from build123d import *

# Parameters (mm, degrees)
F0_R     = 28.2106727932
F0_R_2   = 22.6152096398
F1_DEPTH = 101.6
F3_W     = 56.4213455863
F3_H     = 50.825882433
F4_DEPTH = 3.175


with BuildPart() as f1:
    # F0 (on Top) → F1 (new body)
    with BuildSketch(Plane.XY):
        Circle(F0_R)
        Circle(F0_R_2, mode=Mode.SUBTRACT)
    extrude(amount=F1_DEPTH)


with BuildPart() as f1_1:
    # F2: moved
    add(f1.part.moved(Location((0, 0, -50.8))))

    # F3 (on Top) → F4 (cut)
    with BuildSketch(Plane.XY):
        with Locations((0, 2.7977315767)):
            Rectangle(F3_W, F3_H)
    extrude(amount=F4_DEPTH, mode=Mode.SUBTRACT)


solid = f1_1.part
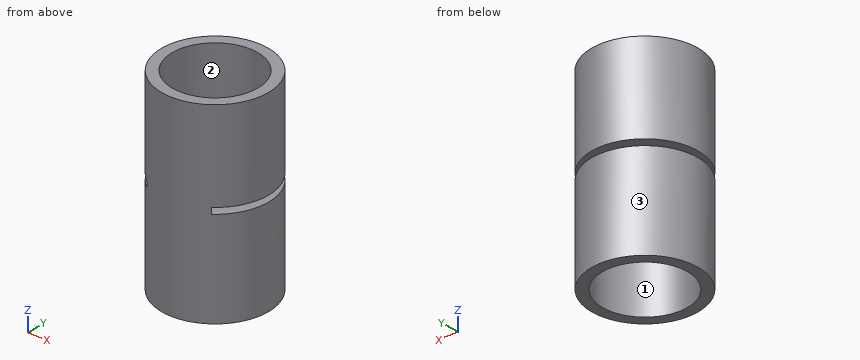
Design review of the part built by this model. Coordinates are the model's own, in mm. Face numbers are marked on the shaded views. Round coordinates to 2 decimals unless told otherwise and drop trailing zeros. Loops run counter-clockwise (first coordinate to the right, second up) from the corner with the lowest first, then second, coordinate; pieces in that order, holes last. Notation, with made-up numbers: (-1.75, 64.5) - (32.25, 64.5) arc R20 ccw to (32.25, 78.5) - close; hole circle Ø5 at (19.5, 89). An arc over 180 degrees is marked (long way). One line per item, written item: value. Start each with the question number.
1) Consider section A-A on y = 0. Give the boundary of the cut face in (x, z) (3 decimals), then the cut area to 3 significant figures.
2) Insertion check: pin 1 Ø4 at (y, z) = (-22, -9.5) entering from +X; pin 2 Ø4 at (x, z) = (-13.5, -33.5) entering from -Y; pin 3 Ø1.5 at (y, z) = (0.5, -12) entering from +X; pin 4 Ø4 at (x, y) = (11.5, 15) entering from +Z. Each pin has a flat end and moves straight along its axis. Give the tip position at first contact, or say it passes through.
3) Consider section C-C on z = 40. Give the boundary of the cut face in (x, y).
4) Consider section D-D on y = 18.5. Give the boundary of the cut face in (x, z) (3 decimals), then the cut area to 3 significant figures.
5) To check wall thickness, follow L1, parallel to X at y = 1, z = -33; L2, parallel to Z at x = 25.5, y = -7 (3 decimals); L3, parallel to Y at x = 0, z = 32. State the ranges of each line that lie inside material, in increasing order. Write a range as from..to.
6) Draft analysis for pull direction Y (two halves, no side actions). For the marked faces 1, 2 and 3, state which applies: +Y half, -Y half, draft (parallel to the pull), parting line (faces both ways), or undercut.
7) Consider section B-B on x = -6. Give the boundary of the cut face in (y, z) (3 decimals).
Reported:
1. outline: (-28.211, -50.8) - (-22.615, -50.8) - (-22.615, 0) - (-28.211, 0) - close; (-28.211, 3.175) - (-22.615, 3.175) - (-22.615, 50.8) - (-28.211, 50.8) - close; (22.615, -50.8) - (28.211, -50.8) - (28.211, 0) - (22.615, 0) - close; (22.615, 3.175) - (28.211, 3.175) - (28.211, 50.8) - (22.615, 50.8) - close
1. area: 1,100 mm^2
2. pin 1: stops at x = 19.9
2. pin 2: stops at y = -25.76
2. pin 3: stops at x = 28.21
2. pin 4: passes through
3. outline: circle Ø56.42 at (0, 0); hole circle Ø45.23 at (0, 0)
4. outline: (-21.298, -50.8) - (-13.008, -50.8) - (-13.008, 0) - (-21.298, 0) - close; (-21.298, 3.175) - (-13.008, 3.175) - (-13.008, 50.8) - (-21.298, 50.8) - close; (13.008, -50.8) - (21.298, -50.8) - (21.298, 0) - (13.008, 0) - close; (13.008, 3.175) - (21.298, 3.175) - (21.298, 50.8) - (13.008, 50.8) - close
4. area: 1,630 mm^2
5. L1: x = -28.19..-22.59, 22.59..28.19
5. L2: z = -50.8..0, 3.175..50.8
5. L3: y = -28.21..-22.62, 22.62..28.21
6. face 1: undercut
6. face 2: undercut
6. face 3: parting line
7. outline: (-27.565, -50.8) - (-21.805, -50.8) - (-21.805, 0) - (-22.615, 0) - (-22.615, 3.175) - (-21.805, 3.175) - (-21.805, 50.8) - (-27.565, 50.8) - close; (21.805, -50.8) - (27.565, -50.8) - (27.565, 0) - (21.805, 0) - close; (21.805, 3.175) - (27.565, 3.175) - (27.565, 50.8) - (21.805, 50.8) - close
